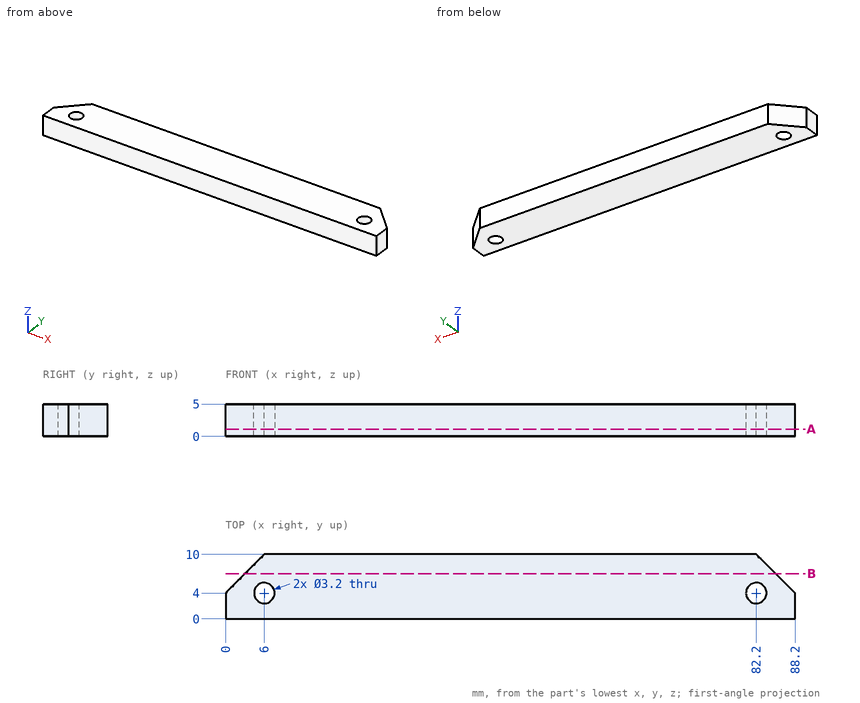
Here's the drawing with two shaded views (mm, measured from the low corner). I have some questions. Give positions to 0.01 mm unless a question says otherwise; leave off trailing zeros. Order: outer loops, then holes, each group sorted by start corner. A loop starts at its lowest first (then second) coordinate and runs counter-clockwise, first axis right, second up.
Q1. I'm going to push a flat-ended pin straight in: P1, Ø4, axis at x = 82.2, y = 4, coming from the +Z side. Where does the tip first touch, or does it pass through?
Q2. Suppose I cut it at A-A, the plane z = 1.1. Write out the boundary of the cut face in (x, y).
Q3. Suppose I cut it at B-B, the plane y = 7. Write out the boundary of the cut face in (x, z).
Q4. If I drill on line 1 along Y through (x, z) = (6, 2.95); line 2 along X through (y, z) = (4.25, 0.6); line 3 along Y through (x, z) = (4, 1.4), over which ranges is the centre line in solid material (lowest first)?
Solution:
1. P1: stops at z = 5
2. outline: (0, 0) - (88.2, 0) - (88.2, 4) - (82.2, 10) - (6, 10) - (0, 4) - close; hole circle Ø3.2 at (6, 4); hole circle Ø3.2 at (82.2, 4)
3. outline: (3, 0) - (85.2, 0) - (85.2, 5) - (3, 5) - close
4. line 1: y = 0 to 2.4, 5.6 to 10
4. line 2: x = 0.25 to 4.42, 7.58 to 80.62, 83.78 to 87.95
4. line 3: y = 0 to 8
